Work out the finished part from the listing and answer in its coordinate system (mm). Face numbers are marked on the shaded views. A direction names the side the tool comes from. Round coordinates to 2 decimals unless told otherwise and drop trailing zeros. Order: outer loops, then holes, each group sorted by start corner. A loop starts at its lowest first (then second) coordinate and runs counter-clockwise, first axis right, second up. Notation, with made-up numbers: (-32, 71.25) - (8, 71.25) arc R4 cw to (8, 75.25) - close; hole circle Ø6 at (-29, 39). An arc over 180 degrees is marked (long way). Put each result on its own line as item: value.
```python
from build123d import *

# Parameters (mm, degrees)
F0_R            = 63.5
F1_DEPTH        = 12.7
F2_R            = 6.35
F3_DEPTH        = 12.701
F5_DEPTH        = 12.701
F5_COPIES_COUNT = 4


# Not quite as in the source:
# - a pattern or mirror of a feature is missing from the dataset's text; its kind, count and spacing are read off the source's solid


with BuildPart() as f1:
    # F0 (on Front) → F1 (new body)
    with BuildSketch(Plane.XZ):
        Circle(F0_R)
    extrude(amount=F1_DEPTH)

    # F2 (on face) → F3 (cut, through all)
    with BuildSketch(Plane.XZ.offset(12.7)):
        Circle(F2_R)
    extrude(amount=-F3_DEPTH, mode=Mode.SUBTRACT)

    # F4 (on face) → F5 (cut, through all)
    with BuildSketch(Plane.XZ.offset(12.7)):
        with BuildLine():
            Line((-22.1979282796, 45.8192452788), (-3.7104284856, 13.9721687883))
            Line((-3.7104284856, 13.9721687883), (3.7104284856, 13.9721687883))
            Line((3.7104284856, 13.9721687883), (22.1979282796, 45.8192452788))
            ThreePointArc((22.1979282796, 45.8192452788), (0, 55.6319138023), (-22.1979282796, 45.8192452788))
        make_face()
    f5 = extrude(amount=-F5_DEPTH, mode=Mode.SUBTRACT)

    # F5_copies: F5 ×4 about axis
    f5_copies_axis = Axis((0, 0, 0), (0, 1, 0))
    for i in range(1, F5_COPIES_COUNT):
        add(f5.rotate(f5_copies_axis, i * 360 / F5_COPIES_COUNT), mode=Mode.SUBTRACT)


solid = f1.part
```
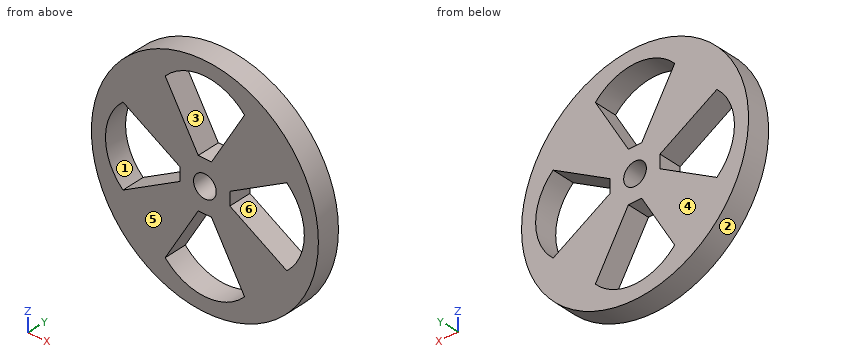
1) For a pull along X with two mould halves and no side action, classify the marked faces 1, 2, 3 and 4 as pulls with the +X half, pulls with the -X half, needs draft (parallel to the pull), parting line crosses it, or undercut.
Findings below:
face 1: undercut
face 2: parting line crosses it
face 3: undercut
face 4: needs draft
2) A cutting plane is placed at B-B on y = -10.5. Write down the section's boundary in (x, z).
Findings below:
outline: circle Ø127 at (0, 0); hole (-45.82, -22.2) - (-13.97, -3.71) - (-13.97, 3.71) - (-45.82, 22.2) arc R30.01 ccw to start; hole (-22.2, -45.82) arc R30.01 ccw to (22.2, -45.82) - (3.71, -13.97) - (-3.71, -13.97) - close; hole (-22.2, 45.82) - (-3.71, 13.97) - (3.71, 13.97) - (22.2, 45.82) arc R30.01 ccw to start; hole circle Ø12.7 at (0, 0); hole (13.97, -3.71) - (45.82, -22.2) arc R30.01 ccw to (45.82, 22.2) - (13.97, 3.71) - close
3) A cutting plane is placed at D-D on z = -34. Write down the section's boundary in (x, y), then the cut area to 3 significant figures.
Findings below:
outline: (-53.63, -12.7) - (-15.34, -12.7) - (-15.34, 0) - (-53.63, 0) - close; (15.34, -12.7) - (53.63, -12.7) - (53.63, 0) - (15.34, 0) - close
area: 973 mm2
4) A cutting plane is placed at A-A on x = 0. Write down the section's boundary in (y, z), then the cut area to 3 significant figures.
Findings below:
outline: (-12.7, -63.5) - (0, -63.5) - (0, -55.63) - (-12.7, -55.63) - close; (-12.7, -13.97) - (0, -13.97) - (0, -6.35) - (-12.7, -6.35) - close; (-12.7, 6.35) - (0, 6.35) - (0, 13.97) - (-12.7, 13.97) - close; (-12.7, 55.63) - (0, 55.63) - (0, 63.5) - (-12.7, 63.5) - close
area: 393 mm2
5) Straight lines are drawn through the part: L1, parallel to X at y = -8.5, z = -17; L2, parallel to Z at x = 19, y = -1.5; L3, parallel to X at y = -9.75, z = -46 (3 decimals). For each, find the intervals that lie inside material, in ascending order. Write a range as from..to.
Findings below:
L1: x = -61.18..-50.35, -36.87..-5.47, 5.47..36.87, 50.35..61.18
L2: z = -60.59..-48.85, -40.31..-6.63, 6.63..40.31, 48.85..60.59
L3: x = -43.775..-22.032, 22.032..43.775
6) A cutting plane is placed at C-C on z = 0. Write down the section's boundary in (x, y), then the cut area to 3 significant figures.
Findings below:
outline: (-63.5, -12.7) - (-55.63, -12.7) - (-55.63, 0) - (-63.5, 0) - close; (-13.97, -12.7) - (-6.35, -12.7) - (-6.35, 0) - (-13.97, 0) - close; (6.35, -12.7) - (13.97, -12.7) - (13.97, 0) - (6.35, 0) - close; (55.63, -12.7) - (63.5, -12.7) - (63.5, 0) - (55.63, 0) - close
area: 393 mm2
7) For the marked faces 5 and 6, determine the directions among +Z, -Z, +X, -X, +Y, -Y from which every point of the face is accessible in a straight line to the end or side of a thin tool.
Findings below:
face 5: +Z, -Z, +X, -X, -Y
face 6: +Y, -Y
8) Given pin 1 Ø2 at (x, y) = (-1.5, -6) entering from -Z; pin 2 Ø11.5 at (x, z) = (0, 0) entering from -Y; pin 3 Ø3 at (y, z) = (-5, 16.5) entering from +X; pin 4 Ø4 at (x, y) = (-21, -2) entering from +Z, each flat-ended and moving along its own axis, determine where each tip first touches the part or whether it passes through.
Findings below:
pin 1: stops at z = -63.5
pin 2: passes through
pin 3: stops at x = 61.7
pin 4: stops at z = 60.59
